Check sheet for the drawn part. Datum: minimum x, y, z corner. Units: mm. A direction names the side the tool comes from. Coordinates: 2 decimals unless noted, no trailing zeros. Write each loop counter-clockwise with the first axis right and the second up, starting at its lowest first coordinate (ties: lowest second). Pieces come first, ordered by that corner, then holes. Notation, with made-up numbers: (61, 61) -> (92, 61) arc R11 cw to (92, 81) -> close; hole circle Ø7 at (-4.75, 40.25). An arc over 180 degrees is marked (long way). One line per question, with ' | ' between items.
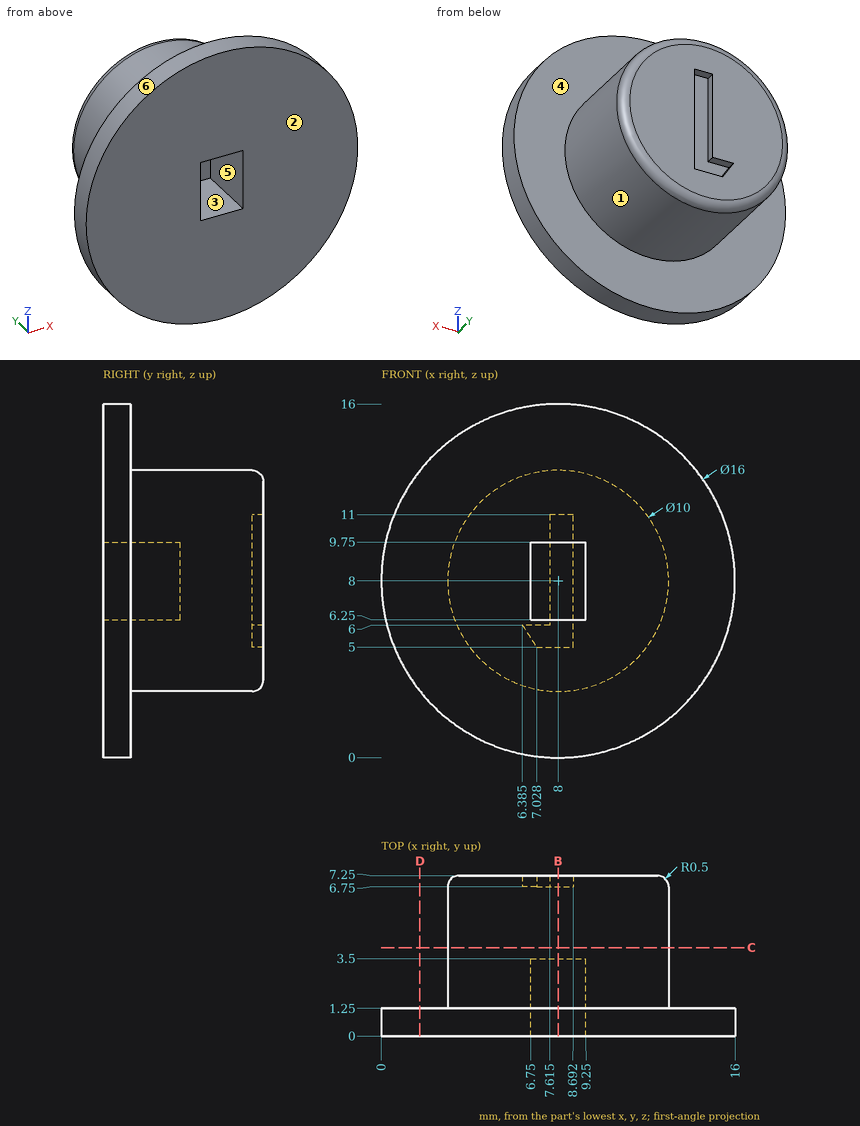
1. Mould release check, pull along X, two halves, no side actions. Record for the marked faces 1, 2 and 3: released by +X, released by -X, zero draft, split by the parting line, or undercut.
Worked answers:
face 1: split by the parting line | face 2: zero draft | face 3: undercut
2. Go/stop test with flat-tipped pins: P1, Ø4, axis at x = 2, z = 3, coming from the +Y side; P2, Ø0.6, axis at x = 8, y = 7, coming from the +Z side; P3, Ø0.6, axis at x = 8, y = 7, coming from the -Z side. Record where each tip stops, or that it passes through.
Worked answers:
P1: y = 1.25 | P2: z = 13 | P3: z = 3
3. Cross-section at B-B on x = 8. Record the boundary of the cut face in (y, z).
Worked answers:
outline: (0, 0) -> (1.25, 0) -> (1.25, 3) -> (6.75, 3) arc R0.5 ccw to (7.25, 3.5) -> (7.25, 5) -> (6.75, 5) -> (6.75, 11) -> (7.25, 11) -> (7.25, 12.5) arc R0.5 ccw to (6.75, 13) -> (1.25, 13) -> (1.25, 16) -> (0, 16) -> (0, 9.75) -> (3.5, 9.75) -> (3.5, 6.25) -> (0, 6.25) -> close
4. Cross-section at D-D on x = 1.75. Record the boundary of the cut face in (y, z).
Worked answers:
outline: (0, 3.01) -> (1.25, 3.01) -> (1.25, 12.99) -> (0, 12.99) -> close
5. Cross-section at C-C on y = 4. Record the boundary of the cut face in (x, z).
Worked answers:
outline: circle Ø10 at (8, 8)
6. Tool access check on the marked faces 4, 5 and 6. Record the directions out of +Z, -Z, +X, -X, +Y, -Y that give a thin tool (end or side, any length) a straight path to the whole face; none if there is none.
Worked answers:
face 4: +Y | face 5: -Y | face 6: +Y, -Y
7. Material ranges on line 1 (X direction, y = 1.75, z = 8); line 2 (Y direction, x = 4.25, z = 1); line 3 (X direction, y = 0.5, z = 6.75), recorded low to high. Write a range as from..to.
Worked answers:
line 1: 3..6.75, 9.25..13 | line 2: 0..1.25 | line 3: 0.1..6.75, 9.25..15.9
